For this review, use the dimensioned drawing (mm, ordinates from the lowest corner) and the shaded views. Coordinates: 2 decimals unless noted, no trailing zeros. Loops run counter-clockwise (first coordinate to the right, second up) from the corner with the lowest first, then second, coordinate; pieces in that order, holes last. Notation, with made-up numbers: (-19.5, 49.5) - (20.5, 49.5) arc R8 ccw to (20.5, 57.5) - close; hole circle Ø7 at (-6.5, 56.5). An arc over 180 degrees is marked (long way). Use one line per item in the form item = value. Start each with the question number.
(1) The part is to be moulded in two halves that separate along Z. For the marked faces 1, 2, 3 and 4, say which applies: pulls with the +Z half, pulls with the -Z half, needs draft (parallel to the pull), parting line crosses it, or undercut.
(2) Add section D-D (z = 46). State the section outline as (x, y) points.
(3) Add section A-A (z = 24). State the section outline as (x, y) points, plus the area to 3 significant figures.
(4) For L1, parallel to Y at x = 10.5, z = 19; L2, parallel to Z at x = 34.5, y = 38.5 (1 decimal); L3, parallel to Z at x = 22, y = 2, list the stretches that pass through material, from the lowest coordinate up.
(5) Add section B-B (x = 22). State the section outline as (y, z) points.
(6) Clearance check with a flat-ended pin moving along its axis: pin 1 Ø16 at (x, z) = (25.52, 25.87) entering from +Y. State where the tip first meets the part, or that it passes through.
(7) Add section C-C (y = 31.5). State the section outline as (x, z) points.
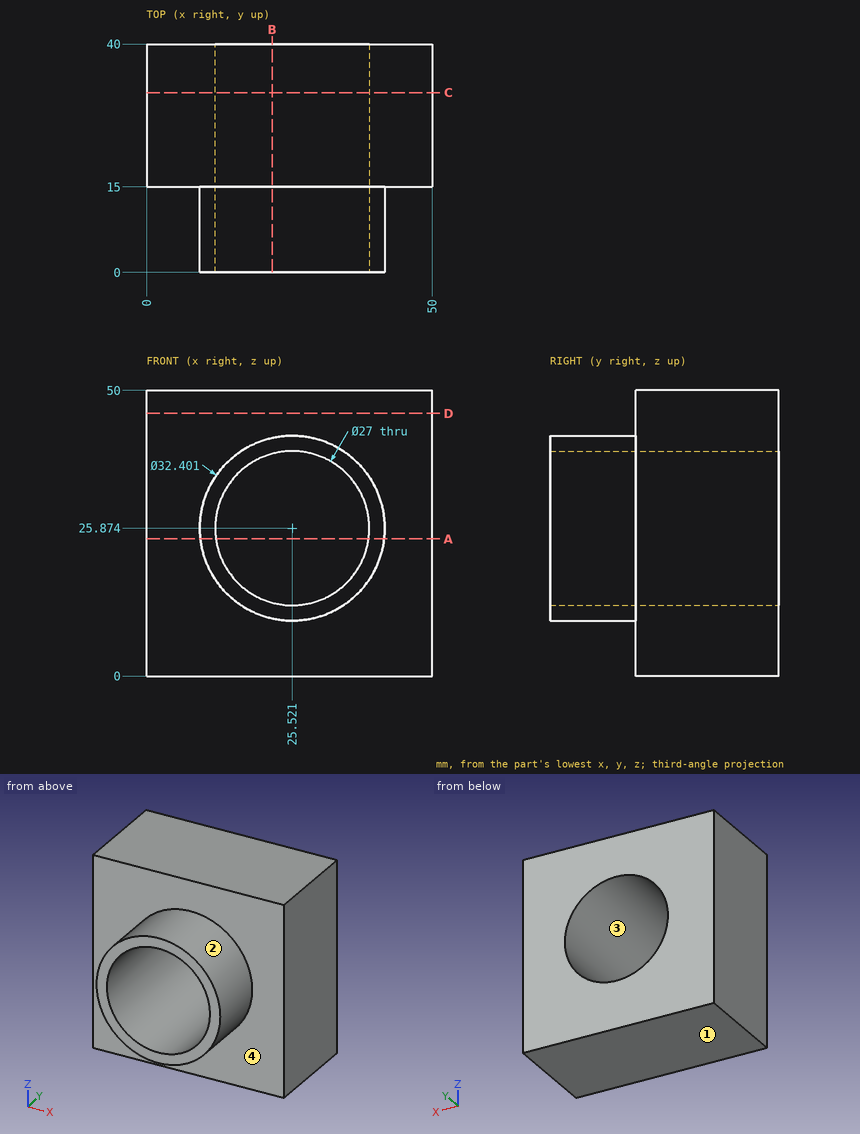
Computed values:
q1.face_1 = pulls with the -Z half
q1.face_2 = parting line crosses it
q1.face_3 = undercut
q1.face_4 = needs draft
q2.outline = (0, 15) - (50, 15) - (50, 40) - (0, 40) - close
q3.outline = (0, 15) - (9.43, 15) - (9.43, 0) - (12.15, 0) - (12.15, 40) - (0, 40) - close; (38.89, 0) - (41.61, 0) - (41.61, 15) - (50, 15) - (50, 40) - (38.89, 40) - close
q3.area = 663 mm^2
q4.L1 = 15 to 40
q4.L2 = 0 to 15.8, 36 to 50
q4.L3 = 10.06 to 12.84, 38.91 to 41.69
q5.outline = (0, 10.06) - (15, 10.06) - (15, 0) - (40, 0) - (40, 12.84) - (0, 12.84) - close; (0, 38.91) - (40, 38.91) - (40, 50) - (15, 50) - (15, 41.69) - (0, 41.69) - close
q6.pin_1 = through
q7.outline = (0, 0) - (50, 0) - (50, 50) - (0, 50) - close; hole circle Ø27 at (25.52, 25.87)
